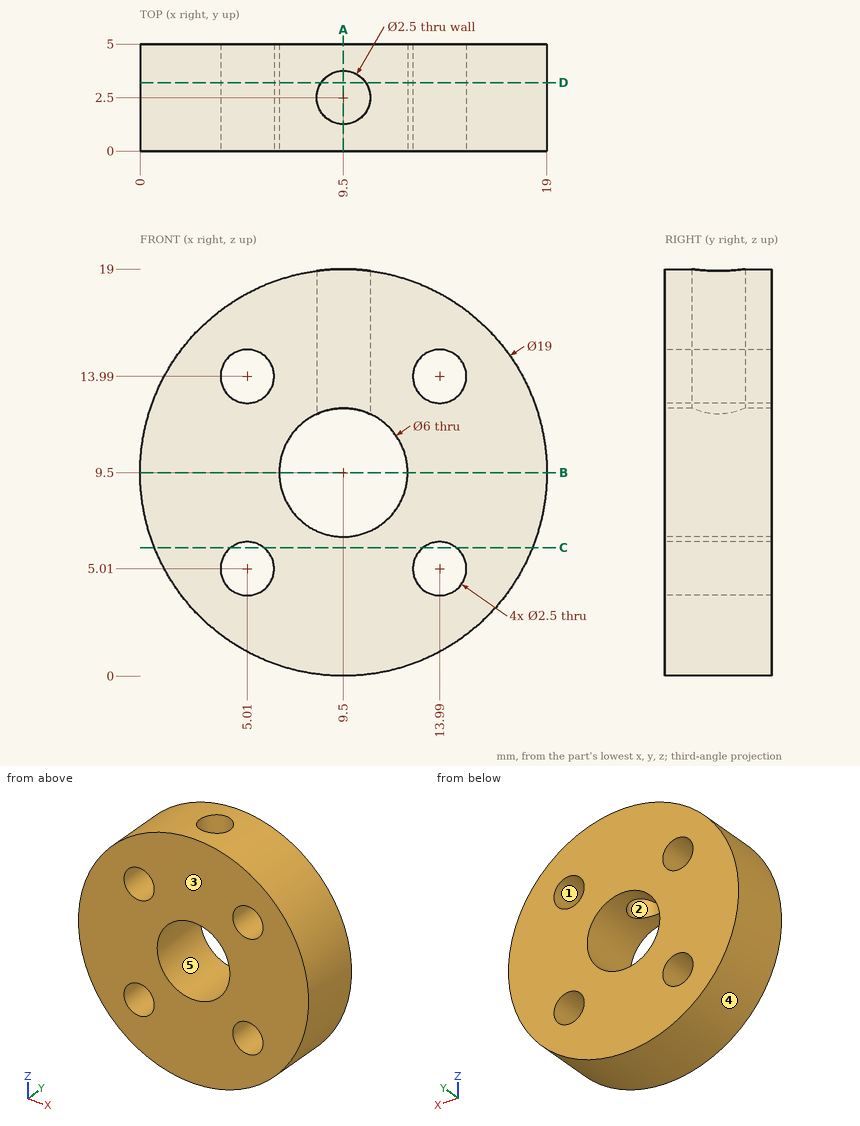
Verification items for this drawing (mm, ordinates from the low corner). A direction names the side the tool comes from. Coordinates: 2 decimals unless noted, no trailing zeros. Loops run counter-clockwise (first coordinate to the right, second up) from the corner with the lowest first, then second, coordinate; pieces in that order, holes last.
Item 1: Sectioned sample at C-C, the plane z = 6. Record the boundary of the cut face in (x, y).
Item 2: Sectioned sample at B-B, the plane z = 9.5. Record the boundary of the cut face in (x, y).
Item 3: Sectioned sample at D-D, the plane y = 3.2. Record the boundary of the cut face in (x, z), then the cut area to 3 significant figures.
Item 4: Access from +Z, -Z, +X, -X, +Y, -Y to the whole of each face (thin tool, end or side, straight path). Record for the marked faces 1 and 2.
Item 5: Sectioned sample at A-A, the plane x = 9.5. Record the boundary of the cut face in (y, z).
Item 6: Go/stop test with flat-tipped pins: pin 1 Ø2 at (x, y) = (6.5, 2) entering from +Z; pin 2 Ø3 at (x, y) = (6.5, 4) entering from -Z; pin 3 Ø3 at (x, z) = (13.99, 13.99) entering from +Y. Record where each tip stops, or that it passes through.
Item 7: Thickness scan on line 1 (Z direction, x = 6, y = 3.85); line 2 (Z direction, x = 13.5, y = 0.6); line 3 (X direction, y = 4.35, z = 5). Record the ranges inside material, lowest first.
Item 8: Release check for a two-part mould opening along Z. For the marked faces 3, 4 and 5 record: released by +Z, released by -Z, zero draft, split by the parting line, or undercut.
Check result:
1. outline: (0.67, 0) - (4.25, 0) - (4.25, 5) - (0.67, 5) - close; (5.77, 0) - (13.23, 0) - (13.23, 5) - (5.77, 5) - close; (14.75, 0) - (18.33, 0) - (18.33, 5) - (14.75, 5) - close
2. outline: (0, 0) - (6.5, 0) - (6.5, 5) - (0, 5) - close; (12.5, 0) - (19, 0) - (19, 5) - (12.5, 5) - close
3. outline: (8.46, 12.32) - (8.46, 18.94) arc R9.5 ccw (long way) to (10.54, 18.94) - (10.54, 12.32) arc R3 cw (long way) to start; hole circle Ø2.5 at (5.01, 5.01); hole circle Ø2.5 at (5.01, 13.99); hole circle Ø2.5 at (13.99, 5.01); hole circle Ø2.5 at (13.99, 13.99)
3. area: 222 mm2
4. face 1: +Y, -Y
4. face 2: +Z
5. outline: (0, 0) - (5, 0) - (5, 6.5) - (0, 6.5) - close; (0, 12.5) - (1.25, 12.5) - (1.25, 19) - (0, 19) - close; (3.75, 12.5) - (5, 12.5) - (5, 19) - (3.75, 19) - close
6. pin 1: stops at z = 18.79
6. pin 2: stops at z = 0.12
6. pin 3: stops at y = 5
7. line 1: z = 0.67 to 4.25, 5.77 to 13.23, 14.75 to 18.33
7. line 2: z = 0.88 to 3.86, 6.16 to 12.84, 15.14 to 18.12
7. line 3: x = 1.13 to 3.76, 6.26 to 12.74, 15.24 to 17.87
8. face 3: zero draft
8. face 4: split by the parting line
8. face 5: undercut
